from build123d import *

# Parameters (mm, degrees)
ESQUISSE1_W             = 110
ESQUISSE1_H             = 68
BOSS_EXTRU_1_DEPTH      = 80
ESQUISSE2_R             = 30
BOSS_EXTRU_2_DEPTH      = 150
CONG_2_R                = 6
ESQUISSE8_R             = 30
ESQUISSE8_R_2           = 15
ENL_V_MAT_EXTRU_1_DEPTH = 35
CONG_3_R                = 6
CONG_4_R                = 10
CONG_5_R                = 10
ENL_V_MAT_EXTRU_2_DEPTH = 10


with BuildPart() as part:
    # Esquisse1 → Boss.-Extru.1 (new body)
    with BuildSketch(Plane.XY):
        with Locations((21.507469619, 14.274916944)):
            Rectangle(ESQUISSE1_W, ESQUISSE1_H)
    extrude(amount=BOSS_EXTRU_1_DEPTH)

    # Esquisse2 → Boss.-Extru.2 (add)
    with BuildSketch(Plane.XY.offset(80)):
        with Locations((46.507469619, 14.274916944)):
            Circle(ESQUISSE2_R)
    extrude(amount=BOSS_EXTRU_2_DEPTH)

    # Congé2
    cong_2_edges = [part.edges().sort_by_distance(p)[0] for p in [
        (16.507469619, 14.274916944, 230),
    ]]
    fillet(cong_2_edges, radius=CONG_2_R)

    # Esquisse8 → Enlèv. mat.-Extru.1 (cut)
    with BuildSketch(Plane.XY.offset(80)):
        with Locations((46.507469619, 14.274916944)):
            Circle(ESQUISSE8_R)
        with Locations((46.507469619, 14.274916944)):
            Circle(ESQUISSE8_R_2, mode=Mode.SUBTRACT)
    extrude(amount=ENL_V_MAT_EXTRU_1_DEPTH, mode=Mode.SUBTRACT)

    # Congé3
    cong_3_edges = [part.edges().sort_by_distance(p)[0] for p in [
        (16.507469619, 14.274916944, 115),
    ]]
    fillet(cong_3_edges, radius=CONG_3_R)

    # Congé4
    cong_4_edges = [part.edges().sort_by_distance(p)[0] for p in [
        (21.507469619, 48.274916944, 80),
        (-33.492530381, 14.274916944, 80),
        (21.507469619, 48.274916944, 0),
        (76.507469619, 14.274916944, 0),
        (21.507469619, -19.725083056, 0),
        (-33.492530381, 14.274916944, 0),
        (21.507469619, -19.725083056, 80),
        (-33.492530381, 48.274916944, 40),
        (76.507469619, 48.274916944, 40),
        (76.507469619, -19.725083056, 40),
        (-33.492530381, -19.725083056, 40),
    ]]
    fillet(cong_4_edges, radius=CONG_4_R)

    # Congé5
    # the kernel refuses this fillet: 10 mm, written as the material it takes off along each edge
    with BuildSketch(Plane(origin=(66.507469619, -9.725083056, 70), x_dir=(1, 0, 0), z_dir=(0, 0, 1))) as cong_5_piece_1_section:
        Polygon((0, 0), (CONG_5_R, 0), (CONG_5_R, -CONG_5_R), (0, -CONG_5_R), align=None)
    cong_5_piece_1 = extrude(amount=CONG_5_R, mode=Mode.PRIVATE)
    cong_5_piece_1 = cong_5_piece_1 - Plane(origin=(66.507469619, -9.725083056, 70), x_dir=(-0.7071067811865475, 0.7071067811865475, 0), z_dir=(0, 0, 1)) * Sphere(CONG_5_R, mode=Mode.PRIVATE)
    add(cong_5_piece_1, mode=Mode.SUBTRACT)
    with BuildSketch(Plane(origin=(66.507469619, 38.274916944, 70), x_dir=(1, 0, 0), z_dir=(0, 0, 1))) as cong_5_piece_2_section:
        Polygon((0, 0), (CONG_5_R, 0), (CONG_5_R, CONG_5_R), (0, CONG_5_R), align=None)
    cong_5_piece_2 = extrude(amount=CONG_5_R, mode=Mode.PRIVATE)
    cong_5_piece_2 = cong_5_piece_2 - Plane(origin=(66.507469619, 38.274916944, 70), x_dir=(-0.7071067811865475, -0.7071067811865475, 0), z_dir=(0, 0, 1)) * Sphere(CONG_5_R, mode=Mode.PRIVATE)
    add(cong_5_piece_2, mode=Mode.SUBTRACT)
    with BuildSketch(Plane(origin=(76.507469619, -9.725083056, 80), x_dir=(-1, 0, 0), z_dir=(0, 1, 0))) as cong_5_piece_3:
        with BuildLine():
            CenterArc((CONG_5_R, -CONG_5_R), CONG_5_R, 90, 90)
            Line((0, -CONG_5_R), (0, 0))
            Line((0, 0), (CONG_5_R, 0))
        make_face()
    extrude(amount=48, mode=Mode.SUBTRACT)

    # Esquisse9 → Enlèv. mat.-Extru.2 (cut)
    with BuildSketch(Plane.XY.offset(80)):
        with BuildLine():
            Line((-18.492530381, 32.274916944), (18.507469619, 32.274916944))
            Line((18.507469619, 32.274916944), (18.507469619, -3.725083056))
            Line((18.507469619, -3.725083056), (-18.492530381, -3.725083056))
            ThreePointArc((-18.492530381, -3.725083056), (-22.028064287, -2.260616962), (-23.492530381, 1.274916944))
            Line((-23.492530381, 1.274916944), (-23.492530381, 27.274916944))
            ThreePointArc((-23.492530381, 27.274916944), (-22.028064287, 30.810450849), (-18.492530381, 32.274916944))
        make_face()
    extrude(amount=-ENL_V_MAT_EXTRU_2_DEPTH, mode=Mode.SUBTRACT)


solid = part.part
Design review of the part built by this model. Coordinates are the model's own, in mm. A direction names the side the tool comes from. Coordinates: 2 decimals unless noted, no trailing zeros. Order: outer loops, then holes, each group sorted by start corner. A loop starts at its lowest first (then second) coordinate and runs counter-clockwise, first axis right, second up. Notation, with made-up numbers: (14.5, 69) -> (40.5, 69) arc R14 cw to (40.5, 91) -> close; hole circle Ø3 at (18.5, -29.5). An arc over 180 degrees is marked (long way). Use one line per item in the form item = value. Start each with the question number.
(1) For probe 1 along Z at (x, y) = (33, 2); probe 2 along Z at (x, y) = (13.5, 23); probe 3 along X at (y, z) = (6, 78.5), list the stretches that pass through material, from the lowest coordinate up.
(2) The part is to be moulded in two halves that separate along Y. For faces 1 (the flat face through (18.507, 15, 75)), 2 (the flat face through (0, -3.725, 75)), 3 (the cylindrical face through (73.656, 45.268, 40.42)), 4 (the cylindrical face through (22.137, -16.718, 77.148)), say which applies: +Y half, -Y half, draft (parallel to the pull), parting line (faces both ways), or undercut.
(3) For faces 5 (the cylindrical face through (35.45, 24.41, 97.26)), 6 (the flat face through (-33.493, 14, 40)), 7 (the cylindrical face through (-21.99, -2.3, 75.07)), 8 (the cylindrical face through (73.5, 13.94, 77.15)), 9 (the cylindrical face through (-30.641, 14.611, 3.007)), list the 3-axis set-ups (+Z, -Z, +X, -X, +Y, -Y) from which the entire face can be reached by the end or side of a thin tool; tool diameter is ignored.
(4) Add section A-A on x = 2. State the section outline as (y, z) points, plus the area to 3 significant figures.
(5) Add section B-B on z = 87. State the section outline as (x, y) points, plus the area to 3 significant figures.
(6) Add section C-C on z = 204.5. State the section outline as (x, y) points, plus the area to 3 significant figures.
(7) Insertion check: pin 1 (5 mm diameter, centred on x = -1.5, z = 74, fed in from +Y); pin 2 (11 mm diameter, centred on x = 1.5, y = 22.5, fed in from +Z); pin 3 (5 mm diameter, centred on y = 23, z = 77, fed in from -X). Each pin has a flat end and moves straight along its axis. Give the tip position at first contact, or say it passes through.
Answer block:
q1.probe_1 = 0 to 80, 115 to 230
q1.probe_2 = 0 to 70
q1.probe_3 = -28.76 to -23.49, 18.51 to 71.78
q2.face_1 = undercut
q2.face_2 = undercut
q2.face_3 = +Y half
q2.face_4 = -Y half
q3.face_5 = none
q3.face_6 = +Z, -Z, -X, +Y, -Y
q3.face_7 = +Z
q3.face_8 = +X, +Y, -Y
q3.face_9 = -Z, -X, +Y, -Y
q4.outline = (-19.73, 10) arc R10 ccw to (-9.73, 0) -> (38.27, 0) arc R10 ccw to (48.27, 10) -> (48.27, 70) arc R10 ccw to (38.27, 80) -> (32.27, 80) -> (32.27, 70) -> (-3.73, 70) -> (-3.73, 80) -> (-9.73, 80) arc R10 ccw to (-19.73, 70) -> close
q4.area = 4,990 mm²
q5.outline = circle Ø30 at (46.51, 14.27)
q5.area = 707 mm²
q6.outline = circle Ø60 at (46.51, 14.27)
q6.area = 2,830 mm²
q7.pin_1 = 48.16
q7.pin_2 = 70
q7.pin_3 = -32.42
